Geometry: see drawing. Coordinates: mm, zero at the bounding-box minimum. Give positions to 0.01 mm unless a question says otherwise; leave off trailing zeros. Order: outer loops, then holes, each group sorted by start corner. A loop starts at its lowest first (then second) coordinate and runs counter-clockwise, first axis right, second up. Notation, with made-up numbers: (14.5, 25) - (32.5, 25) arc R9 ccw to (32.5, 39) - close; hole circle Ø6 at (69.25, -30.75). An arc over 180 degrees is marked (long way). One line per item, written item: value. Start each with the question number.
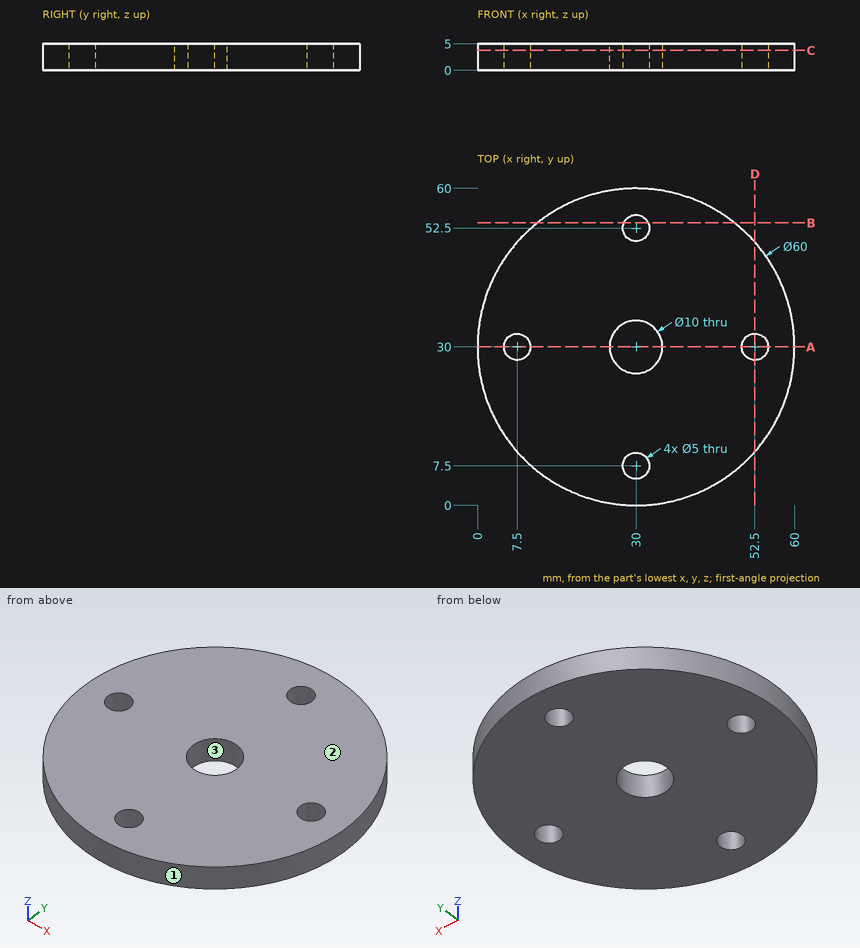
1. Section B-B on y = 53.5. Return the cut outline in (x, z).
2. Section D-D on x = 52.5. Return the cut outline in (y, z), then the cut area to 3 significant figures.
3. Draft query along X for the marked faces 1, 2 and 3. Return one class per face: pulls with the +X half, pulls with the -X half, needs draft (parallel to the pull), parting line crosses it, or undercut.
4. Section A-A on y = 30. Return the cut outline in (x, z), then the cut area to 3 significant figures.
5. Contact query for flat-ended pins moving along their axis: pin 1 Ø2 at (y, z) = (25, 2.5) entering from -X; pin 2 Ø3 at (x, z) = (8.5, 4.5) entering from -Y; pin 3 Ø1 at (y, z) = (28, 4) entering from -X. Output: stop coordinate, or through.
6. Section C-C on z = 3.8. Return the cut outline in (x, y).
7. Ray query, L1, parallel to Y at x = 30, z = 2.95; L2, parallel to Y at x = 32, z = 3.35; L3, parallel to X at y = 30.5, z = 2.35. Return the intervals inside material, ascending.
Data:
1. outline: (11.35, 0) - (27.71, 0) - (27.71, 5) - (11.35, 5) - close; (32.29, 0) - (48.65, 0) - (48.65, 5) - (32.29, 5) - close
2. outline: (10.16, 0) - (27.5, 0) - (27.5, 5) - (10.16, 5) - close; (32.5, 0) - (49.84, 0) - (49.84, 5) - (32.5, 5) - close
2. area: 173 mm2
3. face 1: parting line crosses it
3. face 2: needs draft
3. face 3: undercut
4. outline: (0, 0) - (5, 0) - (5, 5) - (0, 5) - close; (10, 0) - (25, 0) - (25, 5) - (10, 5) - close; (35, 0) - (50, 0) - (50, 5) - (35, 5) - close; (55, 0) - (60, 0) - (60, 5) - (55, 5) - close
4. area: 200 mm2
5. pin 1: stops at x = 0.27
5. pin 2: stops at y = 7.64
5. pin 3: stops at x = 0.04
6. outline: circle Ø60 at (30, 30); hole circle Ø5 at (7.5, 30); hole circle Ø10 at (30, 30); hole circle Ø5 at (30, 7.5); hole circle Ø5 at (30, 52.5); hole circle Ø5 at (52.5, 30)
7. L1: y = 0 to 5, 10 to 25, 35 to 50, 55 to 60
7. L2: y = 0.07 to 6, 9 to 25.42, 34.58 to 51, 54 to 59.93
7. L3: x = 0 to 5.05, 9.95 to 25.03, 34.97 to 50.05, 54.95 to 60
